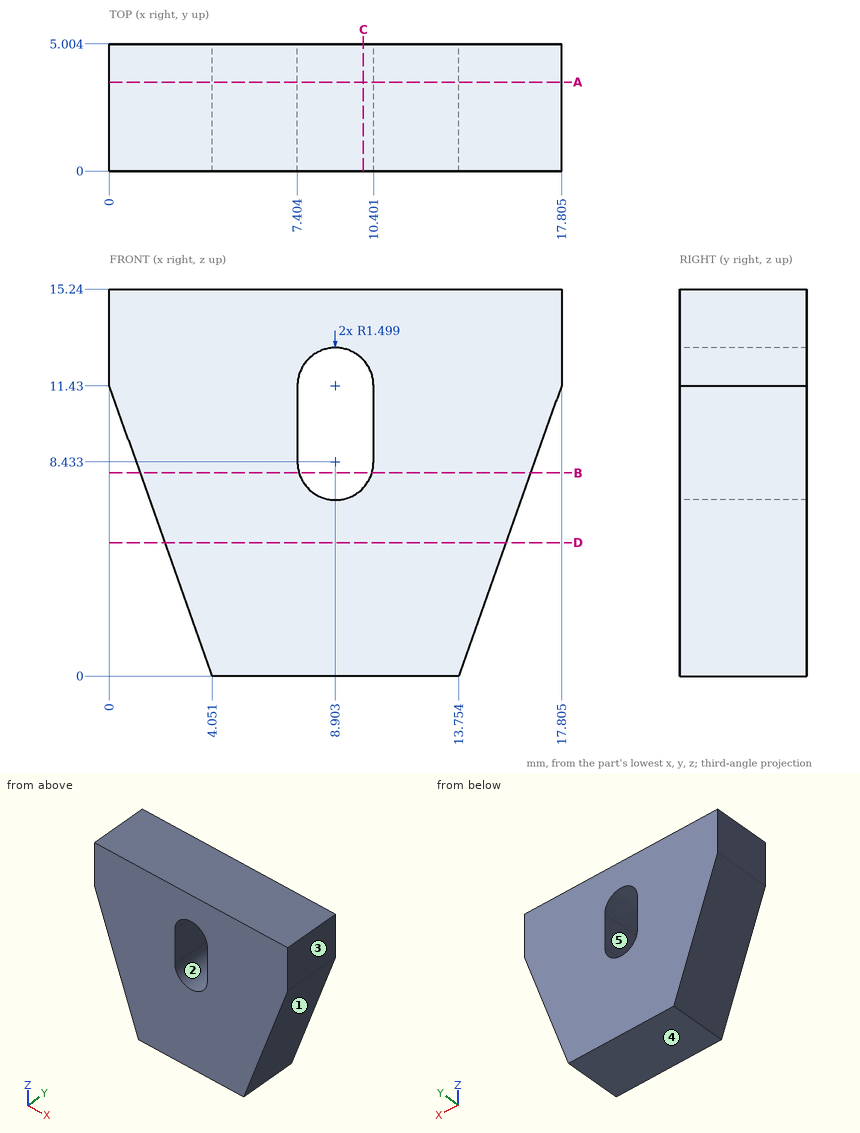
Geometry check sheet. Reference: drawing and pictorial views, mm from the part's lowest x, y, z. A direction names the side the tool comes from. Give positions to 0.01 mm unless a question says otherwise; leave off trailing zeros. Order: outer loops, then holes, each group sorted by start corner. A loop starts at its lowest first (then second) coordinate and runs counter-clockwise, first axis right, second up. Notation, with made-up numbers: M 49,19 L 59,19 A10 ccw 59,33 Z; hole C -12,-30.75 d1. An arc over 180 degrees is marked long. Answer in a Markdown table with one row per item.
1) Cross-section at D-D, the plane z = 5.25. Enter the section's corners in (x, y) (1 decimal).
Filled sheet:
| item | result |
|---|---|
| outline | M 2.2,0 L 15.6,0 L 15.6,5 L 2.2,5 Z |
2) Cross-section at C-C, the plane x = 10. Enter the section's corners in (y, z).
Filled sheet:
| item | result |
|---|---|
| outline | M 0,0 L 5,0 L 5,7.41 L 0,7.41 Z; M 0,12.45 L 5,12.45 L 5,15.24 L 0,15.24 Z |
3) Gauge pin test, flat ends, axial feed: P1, Ø1, axis at y = 3.5, z = 2.5, coming from the +X side; P2, Ø1, axis at y = 0.5, z = 5, coming from the +X side; P3, Ø1.5, axis at y = 3, z = 10.5, coming from the +X side. Record the tip position at first contact, or that the pin passes through.
Filled sheet:
| item | result |
|---|---|
| P1 | stops at x = 14.82 |
| P2 | stops at x = 15.7 |
| P3 | stops at x = 17.74 |
4) Thickness scan on L1, parallel to Z at x = 9, y = 0.8 (1 decimal); L2, parallel to Z at x = 8.5, y = 0.5; L3, parallel to X at y = 4.75, z = 11.25 (1 decimal). Record the ranges inside material, lowest first. Write a range as [from, to].
Filled sheet:
| item | result |
|---|---|
| L1 | z = [0, 6.9], [12.9, 15.2] |
| L2 | z = [0, 6.99], [12.87, 15.24] |
| L3 | x = [0.1, 7.4], [10.4, 17.7] |
5) Release check for a two-part mould opening along Z. For the marked faces 3, 4 and 5 record: +Z half, -Z half, draft (parallel to the pull), parting line (faces both ways), or undercut.
Filled sheet:
| item | result |
|---|---|
| face 3 | draft |
| face 4 | -Z half |
| face 5 | undercut |
6) Access from +Z, -Z, +X, -X, +Y, -Y to the whole of each face (thin tool, end or side, straight path). Record for the marked faces 1 and 2.
Filled sheet:
| item | result |
|---|---|
| face 1 | -Z, +X, +Y, -Y |
| face 2 | +Y, -Y |
7) Cross-section at A-A, the plane y = 3.5. Enter the section's corners in (x, z) (1 decimal), plus the area to 3 significant figures.
Filled sheet:
| item | result |
|---|---|
| outline | M 0,11.4 L 4.1,0 L 13.8,0 L 17.8,11.4 L 17.8,15.2 L 0,15.2 Z; hole M 7.4,8.4 A1.5 ccw 10.4,8.4 L 10.4,11.4 A1.5 ccw 7.4,11.4 Z |
| area | 209 mm2 |
8) Cross-section at B-B, the plane z = 8. Enter the section's corners in (x, y) (1 decimal).
Filled sheet:
| item | result |
|---|---|
| outline | M 1.2,0 L 7.5,0 L 7.5,5 L 1.2,5 Z; M 10.3,0 L 16.6,0 L 16.6,5 L 10.3,5 Z |
